Can you work these out from the model? Positions are in its coordinate system, mm. A direction names the side the tool comes from. Round coordinates to 2 decimals unless told otherwise and drop trailing zeros. Order: outer loops, then holes, each group sorted by start corner. A loop starts at its lowest first (then second) coordinate and runs counter-clockwise, first axis right, second up.
Q1. If we section it at A-A (z = 8.5): Please give me the cut outline in (x, y), plus the area to 3 significant figures.
Q2. If we section it at C-C (y = -16): Please give me the cut outline in (x, z), plus the area to 3 significant figures.
Q3. We'd pull the mould along X, two halves only. Please class faces 4 (the face through (381, 0, 0)), 5 (the face through (189.9, 25.4, -0.2)), 6 (the face through (355.2, 25.4, -0.2)): pulls with the +X half, pulls with the -X half, needs draft (parallel to the pull), parting line crosses it, or undercut.
Q4. Will these pins go through, and if not, where does the flat tip stop? P1, Ø2, axis at x = 317.5, y = -13.5, coming from the +Z side; P2, Ø1, axis at x = 116, z = 9, coming from the +Y side; P3, Ø4, axis at x = 278.5, y = -4, coming from the +Z side.
Q5. If I drill on line 1 (Z direction, x = 28.5, y = -1.5); line 2 (Z direction, x = 88, y = -16.5), over which ranges is the centre line in solid material (lowest first)?
Q6. For faces 1 (the face through (25.8, 25.4, -0.2)), 2 (the face through (303.7, 25.4, -0.2)), 3 (the face through (0, 0, 0)), which set-ups out of +Z, -Z, +X, -X, +Y, -Y let a thin tool reach every point of the face, with its end or its side?
Autodesk Inventor part; units mm, degrees
ref_plane "YZ Plane" through (0, 0, 0) normal (1, 0, 0) x (0, 1, 0)
ref_plane "XZ Plane" through (0, 0, 0) normal (0, 1, 0) x (-1, 0, 0)
ref_plane "XY Plane" through (0, 0, 0) normal (0, 0, 1) x (1, 0, 0)
sketch "Sketch1" plane through (0, 0, 0) normal (0, 0, 1) x (1, 0, 0)
  line L0 (0, 0) -> (381, 0)
  line L1 (0, 0) -> (0, 25.4)
  line L2 (0, 25.4) -> (50.8, 25.4)
  line L3 (50.8, 25.4) -> (50.8, 28.575)
  line L4 (50.8, 28.575) -> (65.786, 28.575)
  line L5 (65.786, 28.575) -> (65.786, 25.4)
  line L6 (65.786, 25.4) -> (86.106, 25.4)
  line L7 (86.106, 25.4) -> (86.106, 28.575)
  line L8 (86.106, 28.575) -> (101.092, 28.575)
  line L9 (101.092, 28.575) -> (101.092, 25.4)
  line L10 (101.092, 25.4) -> (164.592, 25.4)
  line L11 (164.592, 28.575) -> (179.578, 28.575)
  line L12 (179.578, 28.575) -> (179.578, 25.4)
  line L13 (179.578, 25.4) -> (199.898, 25.4)
  line L14 (199.898, 25.4) -> (199.898, 28.575)
  line L15 (199.898, 28.575) -> (214.884, 28.575)
  line L16 (214.884, 28.575) -> (214.884, 25.4)
  line L17 (214.884, 25.4) -> (278.384, 25.4)
  line L18 (278.384, 28.575) -> (293.37, 28.575)
  line L19 (293.37, 28.575) -> (293.37, 25.4)
  line L20 (293.37, 25.4) -> (313.69, 25.4)
  line L21 (313.69, 25.4) -> (313.69, 28.575)
  line L22 (313.69, 28.575) -> (328.676, 28.575)
  line L23 (328.676, 28.575) -> (328.676, 25.4)
  line L24 (328.676, 25.4) -> (379.476, 25.4)
  line L25 (164.592, 28.575) -> (164.592, 25.4)
  line L26 (278.384, 28.575) -> (278.384, 25.4)
  line L27 (379.476, 25.4) -> (381, 25.4)
  line L28 (381, 25.4) -> (381, 0)
  dimension "d0" = 381
  dimension "d1" = 25.4
  dimension "d2" = 50.8
  dimension "d3" = 3.175
  dimension "d4" = 14.986
  dimension "d5" = 20.32
  dimension "d6" = 14.986
  dimension "d7" = 63.5
  dimension "d8" = 14.986
  dimension "d9" = 20.32
  dimension "d10" = 14.986
  dimension "d11" = 63.5
  dimension "d12" = 14.986
  dimension "d13" = 20.32
  dimension "d14" = 14.986
  dimension "d15" = 50.8
revolve "Revolution1" add sketch "Sketch1" angle 360 about axis through (0, 0, 0) along (1, 0, 0)
sketch "Sketch2" plane through (381, 0, 0) normal (1, 0, 0) x (0, 0, -1)
  circle A0 centre (0, 0) radius 28.575
  arc A1 (-12.8501, 21.8127) -> (12.8501, 21.9887) centre (0.1501, -0.0084) ccw
  line L0 (28.575, -0.0084) -> (28.6569, -0.0084) construction
  line L1 (28.5738, -0.2635) -> (28.6458, -0.2635) construction
  line L2 (12.8501, 21.9887) -> (12.8501, 25.5227)
  line L3 (-12.8501, 21.8127) -> (-12.8501, 25.5227)
  line L4 (12.8501, 25.5227) -> (-12.8501, 25.5227)
sketch "Sketch3" plane through (0, 0, 0) normal (-1, 0, 0) x (0, 0, 1)
  circle A0 centre (0, 0) radius 28.575
  arc A1 (-12.7, 21.997) -> (12.7, 21.997) centre (0, 0) ccw
  circle A2 centre (0, 0) radius 28.575
  line L0 (-12.7, 21.997) -> (-12.7, 25.5977)
  line L1 (12.7, 21.997) -> (12.7, 25.5977)
  line L2 (-12.7, 25.5977) -> (12.7, 25.5977)
  dimension "d23" = 57.15
  dimension "d24" = 50.8
extrude "Extrusion1" cut sketch "Sketch3" against normal blind 381 contours A0 L0 A1 L1 | L2 A0
properties part number "Eje"
Solution:
1. outline: (0, -23.94) - (381, -23.94) - (381, 23.94) - (328.68, 23.94) - (328.68, 25.6) - (313.69, 25.6) - (313.69, 23.94) - (293.37, 23.94) - (293.37, 25.6) - (278.38, 25.6) - (278.38, 23.94) - (214.88, 23.94) - (214.88, 25.6) - (199.9, 25.6) - (199.9, 23.94) - (179.58, 23.94) - (179.58, 25.6) - (164.59, 25.6) - (164.59, 23.94) - (101.09, 23.94) - (101.09, 25.6) - (86.11, 25.6) - (86.11, 23.94) - (65.79, 23.94) - (65.79, 25.6) - (50.8, 25.6) - (50.8, 23.94) - (0, 23.94) - close
1. area: 18,400 mm2
2. outline: (0, -19.73) - (381, -19.73) - (381, 19.73) - (0, 19.73) - close
2. area: 15,000 mm2
3. face 4: pulls with the +X half
3. face 5: undercut
3. face 6: needs draft
4. P1: stops at z = 22.11
4. P2: stops at y = 23.94
4. P3: stops at z = 25.32
5. line 1: z = -25.36 to 25.36
5. line 2: z = -19.31 to 19.31
6. face 1: -X, +Y
6. face 2: +Y
6. face 3: +Z, -Z, -X, +Y, -Y
